Could you check a few things on this model? Use its own coordinates, in mm. Give positions to 0.01 mm unless a question says otherwise; leave off trailing zeros. Loops run counter-clockwise (first coordinate to the right, second up) from the corner with the lowest first, then second, coordinate; pieces in that order, holes last. Notation, with made-up numbers: (85.5, 88.5) - (103.5, 88.5) arc R25 cw to (103.5, 111.5) - close; hole circle Ø2 at (-23, 6.25). An arc over 180 degrees is marked (long way). One line per item, written item: value. Start each with the question number.
Q1. I want a section at B-B (x = 36.45). Please give me the cut outline in (y, z).
Q2. If I drill on line 1 (Y direction, x = -36.45, z = 0.7); line 2 (X direction, y = -0.5, z = 0.6); line 3 (X direction, y = 1.25, z = 0.55), over which ranges is the centre line in solid material (lowest first)? Write a range as from..to.
Q3. I want a section at A-A (y = 0). Please give me the cut outline in (x, z) (3 decimals).
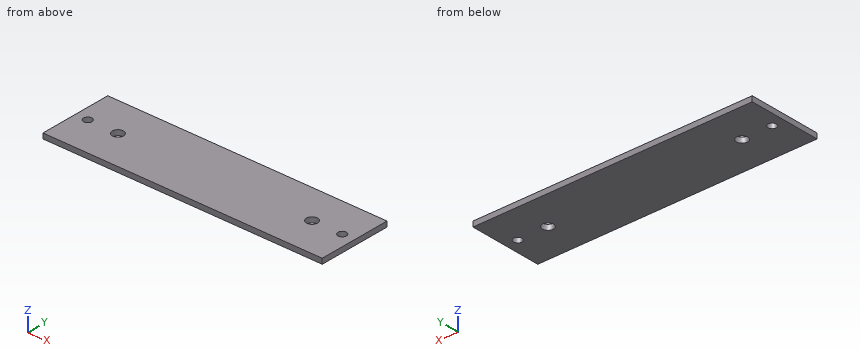
```python
from build123d import *

# Parameters (mm, degrees)
SKETCH1_W           = 80
SKETCH1_H           = 21
SKETCH1_R           = 1.2
SKETCH1_R_2         = 1.6
BOSS_EXTRUDE1_DEPTH = 1.5


with BuildPart() as part:
    # Sketch1 → Boss-Extrude1 (new body)
    with BuildSketch(Plane.XY):
        Rectangle(SKETCH1_W, SKETCH1_H)
        with Locations((-36.45, 0)):
            Circle(SKETCH1_R, mode=Mode.SUBTRACT)
        with Locations((-27.805, 0)):
            Circle(SKETCH1_R_2, mode=Mode.SUBTRACT)
        with Locations(Location((27.805, 0, 0), (0, 0, 180))):
            Circle(SKETCH1_R_2, mode=Mode.SUBTRACT)
        with Locations(Location((36.45, 0, 0), (0, 0, 180))):
            Circle(SKETCH1_R, mode=Mode.SUBTRACT)
    extrude(amount=BOSS_EXTRUDE1_DEPTH)


solid = part.part
```
Worked answers:
1. outline: (-10.5, 0) - (-1.2, 0) - (-1.2, 1.5) - (-10.5, 1.5) - close; (1.2, 0) - (10.5, 0) - (10.5, 1.5) - (1.2, 1.5) - close
2. line 1: y = -10.5..-1.2, 1.2..10.5
2. line 2: x = -40..-37.54, -35.36..-29.32, -26.29..26.29, 29.32..35.36, 37.54..40
2. line 3: x = -40..-28.8, -26.81..26.81, 28.8..40
3. outline: (-40, 0) - (-37.65, 0) - (-37.65, 1.5) - (-40, 1.5) - close; (-35.25, 0) - (-29.405, 0) - (-29.405, 1.5) - (-35.25, 1.5) - close; (-26.205, 0) - (26.205, 0) - (26.205, 1.5) - (-26.205, 1.5) - close; (29.405, 0) - (35.25, 0) - (35.25, 1.5) - (29.405, 1.5) - close; (37.65, 0) - (40, 0) - (40, 1.5) - (37.65, 1.5) - close
